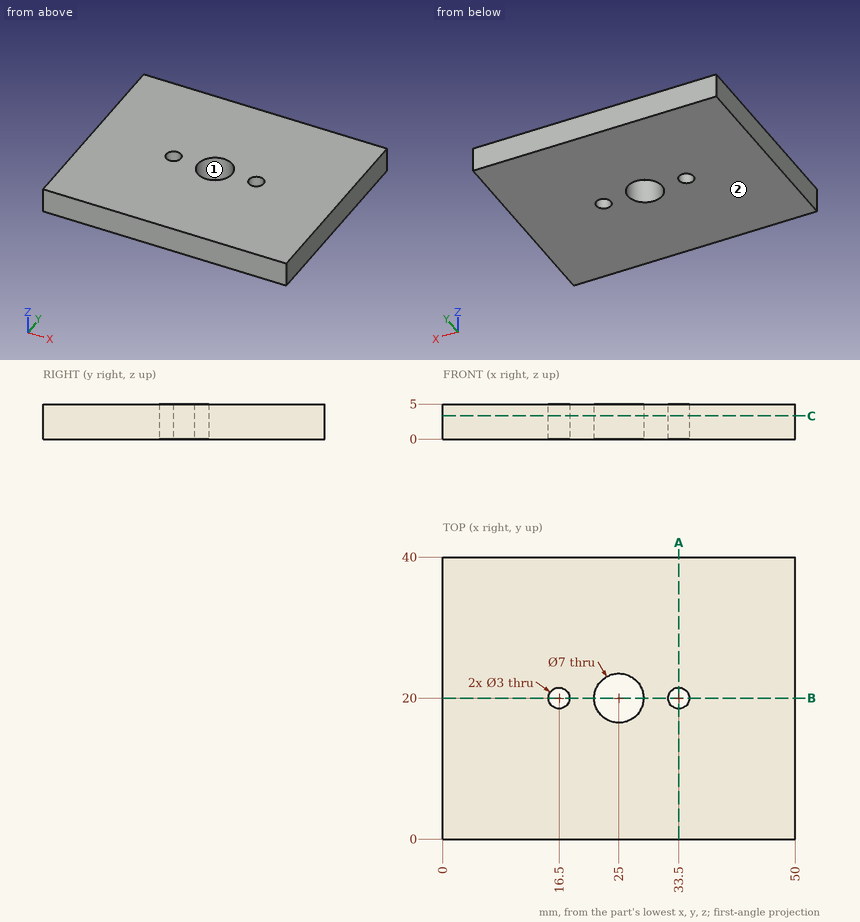
Source: three-view drawing plus pictorial views. Frame: mm from the lowest corner of the part. Give positions to 0.01 mm unless a question says otherwise; leave off trailing zeros. Loops run counter-clockwise (first coordinate to the right, second up) from the corner with the lowest first, then second, coordinate; pieces in that order, holes last. Notation, with made-up numbers: (52.25, 38.25) -> (99.25, 38.25) arc R23 ccw to (99.25, 76.25) -> close; hole circle Ø1 at (61, 30.25). An arc over 180 degrees is marked (long way). Put each result on its own line as item: value. Start each with the question number.
1) Cut plane A-A (x = 33.5). Return loops of the section in (y, z).
2) Cut plane C-C (z = 3.3). Return loops of the section in (x, y).
3) Cut plane B-B (y = 20). Return loops of the section in (x, z), then the cut area to 3 significant figures.
4) Draft query along X for the marked faces 1 and 2. Return one class per face: released by +X, released by -X, zero draft, split by the parting line, or undercut.
5) Material intervals for probe 1 along Y at (x, z) = (33.5, 2.7); probe 2 along Y at (x, z) = (25, 3.4); probe 3 along X at (y, z) = (22, 0.8), sorted ascending.
6) Contact query for a flat-ended pin moving along its axis: P1, Ø2.5, axis at x = 16.5, y = 20, coming from the -Z side. Output: stop coordinate, or through.
Results are:
1. outline: (0, 0) -> (18.5, 0) -> (18.5, 5) -> (0, 5) -> close; (21.5, 0) -> (40, 0) -> (40, 5) -> (21.5, 5) -> close
2. outline: (0, 0) -> (50, 0) -> (50, 40) -> (0, 40) -> close; hole circle Ø3 at (16.5, 20); hole circle Ø7 at (25, 20); hole circle Ø3 at (33.5, 20)
3. outline: (0, 0) -> (15, 0) -> (15, 5) -> (0, 5) -> close; (18, 0) -> (21.5, 0) -> (21.5, 5) -> (18, 5) -> close; (28.5, 0) -> (32, 0) -> (32, 5) -> (28.5, 5) -> close; (35, 0) -> (50, 0) -> (50, 5) -> (35, 5) -> close
3. area: 185 mm2
4. face 1: undercut
4. face 2: zero draft
5. probe 1: y = 0 to 18.5, 21.5 to 40
5. probe 2: y = 0 to 16.5, 23.5 to 40
5. probe 3: x = 0 to 22.13, 27.87 to 50
6. P1: passes through
